Can you work these out from the model? Positions are in its coordinate system, mm. A direction names the side the tool comes from. Coordinates: 2 decimals unless noted, no trailing zeros. Order: outer loops, then holes, each group sorted by start corner. A loop starts at its lowest first (then second) coordinate and runs counter-clockwise, first axis right, second up. Notation, with made-up numbers: (23, -37) -> (27, -37) arc R23 ccw to (27, -11) -> close; hole circle Ø11 at (-21, 74). An arc over 180 degrees is marked (long way). Write item = value, one per line.
```python
from build123d import *

# Parameters (mm, degrees)
SKETCH_1_W           = 30
SKETCH_1_H           = 28
EXTRUDE_1_DEPTH      = 10
CUT_EXTRUDE_2_DEPTH  = 0.8
M1_4X0_3_2_D         = 1.1
M1_4X0_3_2_DEPTH     = 3.7
M1_4X0_3_2_TIP       = 0.33047334
CUT_EXTRUDE_4_DEPTH  = 0.5
SKETCH_12_W          = 30
SKETCH_12_H          = 4.25
CUT_EXTRUDE_5_DEPTH  = 10
SKETCH_13_R          = 1.7
CUT_EXTRUDE_6_DEPTH  = 10
SKETCH_14_W          = 23
SKETCH_14_H          = 23.75
CUT_EXTRUDE_7_DEPTH  = 5
CUT_EXTRUDE_9_DEPTH  = 3
SKETCH_20_W          = 7
SKETCH_20_H          = 23.75
SKETCH_20_R          = 1.7
EXTRUDE_3_DEPTH      = 4.1
SKETCH_23_W          = 4
SKETCH_23_H          = 23.75
EXTRUDE_4_DEPTH      = 9.1
SKETCH_24_W          = 16.2
SKETCH_24_H          = 4.1
CUT_EXTRUDE_10_DEPTH = 5
SKETCH_29_W          = 16.2
SKETCH_29_H          = 2
EXTRUDE_5_DEPTH      = 4.1
SKETCH_30_R          = 1.15
SKETCH_30_R_2        = 0.6
CUT_EXTRUDE_12_DEPTH = 5


with BuildPart() as part:
    # 草图1 → 凸台-拉伸1 (new body)
    with BuildSketch(Plane.XY):
        with Locations((7.449728974, 2.736434109)):
            Rectangle(SKETCH_1_W, SKETCH_1_H)
    extrude(amount=EXTRUDE_1_DEPTH)

    # 草图2 → 切除-拉伸2 (cut)
    with BuildSketch(Plane(origin=(0, 0, 0), x_dir=(-1, 0, 0), z_dir=(0, 0, -1))):
        with BuildLine():
            Line((5.050271026, 16.736434109), (-15.449728974, 16.736434109))
            Line((-15.449728974, 16.736434109), (-15.449728974, 3.736434109))
            ThreePointArc((-15.449728974, 3.736434109), (-14.571049317, 1.615113765), (-12.449728974, 0.736434109))
            Line((-12.449728974, 0.736434109), (2.050271026, 0.736434109))
            ThreePointArc((2.050271026, 0.736434109), (4.17159137, 1.615113765), (5.050271026, 3.736434109))
            Line((5.050271026, 3.736434109), (5.050271026, 16.736434109))
        make_face()
    extrude(amount=-CUT_EXTRUDE_2_DEPTH, mode=Mode.SUBTRACT)

    # M1.4x0.3 螺纹孔2
    with Locations(Plane(origin=(0, 0, 0.8), x_dir=(-1, 0, 0), z_dir=(0, 0, -1))):
        with Locations((-12.199728974, 8.736434109), (1.800271026, 8.736434109)):
            Hole(M1_4X0_3_2_D / 2, depth=M1_4X0_3_2_DEPTH)
            with Locations((0, 0, -(M1_4X0_3_2_DEPTH + M1_4X0_3_2_TIP / 2))):  # 118° drill point
                Cone(0, M1_4X0_3_2_D / 2, M1_4X0_3_2_TIP, mode=Mode.SUBTRACT)

    # 草图11 → 切除-拉伸4 (cut)
    with BuildSketch(Plane(origin=(0, 0, 0), x_dir=(-1, 0, 0), z_dir=(0, 0, -1))):
        with BuildLine():
            Line((-7.549728974, -2.063565891), (-2.849728974, -2.063565891))
            ThreePointArc((-2.849728974, -2.063565891), (-2.422952278, -2.240342587), (-2.599728974, -1.813565891))
            Line((-2.599728974, -1.813565891), (-2.599728974, 0.736434109))
            Line((-2.599728974, 0.736434109), (-7.799728974, 0.736434109))
            Line((-7.799728974, 0.736434109), (-7.799728974, -1.813565891))
            ThreePointArc((-7.799728974, -1.813565891), (-7.976505669, -2.240342587), (-7.549728974, -2.063565891))
        make_face()
    extrude(amount=-CUT_EXTRUDE_4_DEPTH, mode=Mode.SUBTRACT)

    # 草图12 → 切除-拉伸5 (cut)
    with BuildSketch(Plane(origin=(0, 0, 0), x_dir=(-1, 0, 0), z_dir=(0, 0, -1))):
        with Locations((-7.449728974, -9.138565891)):
            Rectangle(SKETCH_12_W, SKETCH_12_H)
    extrude(amount=-CUT_EXTRUDE_5_DEPTH, mode=Mode.SUBTRACT)

    # 草图13 → 切除-拉伸6 (cut)
    with BuildSketch(Plane(origin=(0, 0, 0), x_dir=(-1, 0, 0), z_dir=(0, 0, -1))):
        with Locations((-18.199728974, 9.686434109)):
            Circle(SKETCH_13_R)
    extrude(amount=-CUT_EXTRUDE_6_DEPTH, mode=Mode.SUBTRACT)

    # 草图14 → 切除-拉伸7 (cut)
    with BuildSketch(Plane.XY.offset(10)):
        with Locations((3.949728974, 4.861434109)):
            Rectangle(SKETCH_14_W, SKETCH_14_H)
    extrude(amount=-CUT_EXTRUDE_7_DEPTH, mode=Mode.SUBTRACT)

    # 草图16 → 切除-拉伸9 (cut)
    with BuildSketch(Plane.XY.offset(5)):
        with BuildLine():
            Line((-1.300271026, -7.013565891), (11.699728974, -7.013565891))
            Line((11.699728974, -7.013565891), (11.699728974, -0.513565891))
            ThreePointArc((11.699728974, -0.513565891), (5.199728974, 5.986434109), (-1.300271026, -0.513565891))
            Line((-1.300271026, -0.513565891), (-1.300271026, -7.013565891))
        make_face()
    extrude(amount=-CUT_EXTRUDE_9_DEPTH, mode=Mode.SUBTRACT)

    # 草图20 → 凸台-拉伸3 (add)
    with BuildSketch(Plane.XY.offset(10)):
        with Locations((18.949728974, 4.861434109)):
            Rectangle(SKETCH_20_W, SKETCH_20_H)
        with Locations(Location((18.199728974, 9.686434109, 0), (0, 0, 180))):
            Circle(SKETCH_20_R, mode=Mode.SUBTRACT)
    extrude(amount=EXTRUDE_3_DEPTH)

    # 草图23 → 凸台-拉伸4 (add)
    with BuildSketch(Plane.XY.offset(5)):
        with Locations((-5.550271026, 4.861434109)):
            Rectangle(SKETCH_23_W, SKETCH_23_H)
    extrude(amount=EXTRUDE_4_DEPTH)

    # 草图24 → 切除-拉伸10 (cut)
    with BuildSketch(Plane(origin=(0, 0, 0.8), x_dir=(-1, 0, 0), z_dir=(0, 0, -1))):
        with Locations((-5.199728974, 14.686434109)):
            Rectangle(SKETCH_24_W, SKETCH_24_H)
    extrude(amount=-CUT_EXTRUDE_10_DEPTH, mode=Mode.SUBTRACT)

    # 草图29 → 凸台-拉伸5 (add)
    with BuildSketch(Plane(origin=(0, 12.636434109, 0), x_dir=(1, 0, 0), z_dir=(0, 1, 0))):
        with Locations((5.199728974, -1.8)):
            Rectangle(SKETCH_29_W, SKETCH_29_H)
    extrude(amount=EXTRUDE_5_DEPTH)

    # 草图30 → 切除-拉伸12 (cut)
    with BuildSketch(Plane(origin=(0, 0, 0.8), x_dir=(-1, 0, 0), z_dir=(0, 0, -1))):
        with Locations((0.900271026, 14.736434109)):
            Circle(SKETCH_30_R)
        with Locations((-11.299728974, 14.736434109)):
            Circle(SKETCH_30_R)
        with Locations((-1.449728974, 14.736434109)):
            Circle(SKETCH_30_R_2)
        with Locations((-8.949728974, 14.736434109)):
            Circle(SKETCH_30_R_2)
    extrude(amount=-CUT_EXTRUDE_12_DEPTH, mode=Mode.SUBTRACT)


solid = part.part
```
Item 1: If I drill on probe 1 along X at (y, z) = (15.25, 3.5); probe 2 along X at (y, z) = (6.5, 11.5); probe 3 along Z at (x, y) = (5.25, 10), over which ranges is the centre line in solid material (lowest first)?
A:
probe_1 = -7.55 to -2.9, 13.3 to 22.45
probe_2 = -7.55 to -3.55, 15.45 to 22.45
probe_3 = 0.8 to 5
Item 2: I'm going to push flat-ended pins straight in: P1, Ø5.5, axis at x = 5, y = 3.5, coming from the +Z side; P2, Ø6, axis at x = 8.5, z = 8.5, coming from the -Y side; P3, Ø10, axis at x = 4.5, y = -4.5, coming from the +Z side; P4, Ø0.6, axis at x = 6, z = 0, coming from the +Y side. Where does each tip first touch, or does it pass through?
A:
P1 = 5
P2 = through
P3 = 2
P4 = -2.06
Item 3: I want a section at D-D, the plane x = 5.5. Please give me the cut outline in (y, z), plus the area to 3 significant figures.
A:
outline = (-7.01, 0) -> (-2.06, 0) -> (-2.06, 0.5) -> (0.74, 0.5) -> (0.74, 0.8) -> (16.74, 0.8) -> (16.74, 2.8) -> (12.64, 2.8) -> (12.64, 5) -> (5.98, 5) -> (5.98, 2) -> (-7.01, 2) -> close
area = 56.6 mm2
Item 4: If we mould it in two halves opening along Y, with no side actions, what happens to faces 1 (the flat face through (8, 8, 5)), 2 (the cylindrical face through (5.343, 5.985, 3.521)), 3 (the cylindrical face through (-0.651, 13.614, 1.786))? For each: pulls with the +Y half, pulls with the -Y half, needs draft (parallel to the pull), parting line crosses it, or undercut.
A:
face_1 = needs draft
face_2 = pulls with the -Y half
face_3 = undercut
Item 5: I want a section at A-A, the plane x = 8.75. Please give me the cut outline in (y, z), plus the area to 3 significant figures.
A:
outline = (-7.01, 0) -> (0.74, 0) -> (0.74, 0.8) -> (14.17, 0.8) -> (14.17, 2.8) -> (12.64, 2.8) -> (12.64, 5) -> (4.93, 5) -> (4.93, 2) -> (-7.01, 2) -> close; (15.3, 0.8) -> (16.74, 0.8) -> (16.74, 2.8) -> (15.3, 2.8) -> close
area = 58.8 mm2
Item 6: I want a section at B-B, the plane z = 6.25. Please give me the cut outline in (x, y).
A:
outline = (-7.55, -7.01) -> (-3.55, -7.01) -> (-3.55, 16.74) -> (-7.55, 16.74) -> close; (15.45, -7.01) -> (22.45, -7.01) -> (22.45, 16.74) -> (15.45, 16.74) -> close; hole circle Ø3.4 at (18.2, 9.69)
Item 7: For faces 4 (the cylindrical face through (11.763, 8.402, 2.676)), 5 (the flat face through (5, 12.636, 4)), 6 (the flat face through (-1.3, -4, 4)), 7 (the flat face through (5, 9, 0.8)), which set-ups out of +Z, -Z, +X, -X, +Y, -Y let a thin tool reach every point of the face, with its end or its side?
A:
face_4 = -Z
face_5 = +Z, +Y
face_6 = +Z, -Y
face_7 = -Z, +Y
Item 8: I want a section at C-C, the plane y = -4.5. Please give me the cut outline in (x, z).
A:
outline = (-7.55, 0) -> (22.45, 0) -> (22.45, 14.1) -> (15.45, 14.1) -> (15.45, 5) -> (11.7, 5) -> (11.7, 2) -> (-1.3, 2) -> (-1.3, 5) -> (-3.55, 5) -> (-3.55, 14.1) -> (-7.55, 14.1) -> close
